Read the model definition and answer for the solid it produces. Units are mm, in the model's axes. A direction names the side the tool comes from. Round coordinates to 2 decimals unless told otherwise and drop trailing zeros. Order: outer loops, then holes, each group sorted by start corner. A loop starts at its lowest first (then second) coordinate and runs counter-clockwise, first axis right, second up. Notation, with made-up numbers: (-31.75, 49) - (5.25, 49) arc R22 cw to (5.25, 81) - close; hole circle Ø9 at (12.25, 43). An arc over 180 degrees is marked (long way). Put each result on its own line as item: value. Start each with the question number.
Q1. Section C-C on z = 36 is taken. Give the vertices of the cut face in (x, y).
Q2. Find the intervals of material crossed by line 1 along Y through (x, z) = (-19, 1.6); line 2 along X through (y, z) = (-7, 123); line 3 along X through (y, z) = (-7.25, 114.5), in increasing order. Write a range as from..to.
Q3. Each of these flat-tipped pins is pushed along its axis until it touches: pin 1 Ø9 at (y, z) = (-13, 81.5) entering from +X; pin 2 Ø5.5 at (x, z) = (0, 51.5) entering from +Y; pin 3 Ø1.5 at (x, y) = (-11, -15.5) entering from +Z; pin 4 Ø2.5 at (x, y) = (-19, -15) entering from -Z. Where does it stop, or does it pass through?
Q4. Which of the six approach directions +Z, -Z, +X, -X, +Y, -Y give full straight-line access (tool end or side, diameter ignored) to faces 1 (the face through (-9, -15, 6)), 2 (the face through (-0.05, -21.45, 100.94))?
Q5. Section B-B on y = -1.75 is taken. Give the vertices of the cut face in (x, z), then the cut area to 3 significant figures.
Q6. For a pull along X with two mould halves and no side action, classify faces 3 (the face through (9, -15, 7)), 4 (the face through (0, -14.279, 85)), 5 (the face through (1.85, -14.79, 126.33)) as pulls with the +X half, pulls with the -X half, needs draft (parallel to the pull), parting line crosses it, or undercut.
Q7. Section A-A on x = -19 is taken. Give the vertices of the cut face in (y, z).
Q8. Section D-D on x = 0 is taken. State how many separate pieces and enclosed holes the cut face has, then the cut area to 3 significant figures.
from build123d import *

# Parameters (mm, degrees)
F0_R     = 3.45
F1_DEPTH = 30
F2_R     = 1.5
F3_DEPTH = 25.4
F5_DEPTH = 25.4


with BuildPart() as f1:
    # F0 (on Front) → F1 (new body)
    with BuildSketch(Plane.XZ):
        Polygon((-24, 5), (-24, 0), (-9, 0), (-9, 13), (0, 13), (9, 13), (9, 0), (24, 0), (24, 5), (14, 5), (14, 18), (10.571068, 18), (3.5, 18), (0, 18), (-3.5, 18), (-10.571068, 18), (-14, 18), (-14, 5), align=None)
        Polygon((-3.5, 25.071068), (-10.571068, 18), (-3.5, 18), align=None)
        with BuildLine():
            Line((-3.5, 25.071068), (-3.5, 18))
            Line((-3.5, 18), (0, 18))
            Line((0, 18), (3.5, 18))
            Line((3.5, 18), (3.5, 25.071068))
            Line((3.5, 25.071068), (3.5, 118))
            ThreePointArc((3.5, 118), (0, 116.967795), (-3.5, 118))
            Line((-3.5, 118), (-3.5, 25.071068))
        make_face()
        with BuildLine():
            ThreePointArc((6.45, 123.417795), (-3.084437, 129.082488), (-3.5, 118))
            ThreePointArc((-3.5, 118), (0, 116.967795), (3.5, 118))
            ThreePointArc((3.5, 118), (5.664693, 120.333358), (6.45, 123.417795))
        make_face()
        with Locations((0, 123.417795)):
            Circle(F0_R, mode=Mode.SUBTRACT)
        Polygon((3.5, 25.071068), (3.5, 18), (10.571068, 18), align=None)
    extrude(amount=F1_DEPTH)

    # F2 (on face) → F3 (cut)
    with BuildSketch(Plane.XY.offset(5)):
        with Locations((19, -15)):
            Circle(F2_R)
        with Locations((-19, -15)):
            Circle(F2_R)
    extrude(amount=-F3_DEPTH, mode=Mode.SUBTRACT)

    # F4 (on face) → F5 (cut)
    with BuildSketch(Plane(origin=(-3.5, 0, 0), x_dir=(0, -1, 0), z_dir=(-1, 0, 0))):
        Polygon((14.351341, 41.974204), (4.138201, 34.047591), (14.351341, 34.047591), align=None)
        Polygon((4.138201, 38.620638), (14.351341, 46.547251), (4.138201, 46.852125), align=None)
        Polygon((14.351341, 57.451731), (4.138201, 49.525118), (14.351341, 49.525118), align=None)
        Polygon((4.138201, 54.098165), (14.351341, 62.024778), (4.138201, 62.329652), align=None)
        Polygon((14.279029, 73.874906), (4.065889, 65.948293), (14.279029, 65.948293), align=None)
        Polygon((4.065889, 70.52134), (14.279029, 78.447953), (4.065889, 78.752828), align=None)
        Polygon((14.279029, 89.352433), (4.065889, 81.42582), (14.279029, 81.42582), align=None)
        Polygon((4.065889, 85.998867), (14.279029, 93.92548), (4.065889, 94.230354), align=None)
        Polygon((26.558967, 41.64265), (16.345827, 33.716037), (26.558967, 33.716037), align=None)
        Polygon((16.345827, 38.289084), (26.558967, 46.215698), (16.345827, 46.520572), align=None)
        Polygon((26.558967, 57.120177), (16.345827, 49.193564), (26.558967, 49.193564), align=None)
        Polygon((16.345827, 53.766611), (26.558967, 61.693224), (16.345827, 61.998098), align=None)
        Polygon((26.486655, 73.543353), (16.273515, 65.61674), (26.486655, 65.61674), align=None)
        Polygon((16.273515, 70.189787), (26.486655, 78.1164), (16.273515, 78.421274), align=None)
        Polygon((26.486655, 89.02088), (16.273515, 81.094267), (26.486655, 81.094267), align=None)
        Polygon((16.273515, 85.667314), (26.486655, 93.593927), (16.273515, 93.898801), align=None)
        Polygon((14.279029, 105.178627), (4.065889, 97.252014), (14.279029, 97.252014), align=None)
        Polygon((4.065889, 101.825062), (14.279029, 109.751675), (4.065889, 110.056549), align=None)
        Polygon((26.486655, 104.847074), (16.273515, 96.920461), (26.486655, 96.920461), align=None)
        Polygon((16.273515, 101.493508), (26.486655, 109.420121), (16.273515, 109.724995), align=None)
    extrude(amount=-F5_DEPTH, mode=Mode.SUBTRACT)


solid = f1.part
Findings:
1. outline: (-3.5, -30) - (3.5, -30) - (3.5, -26.56) - (-3.5, -26.56) - close; (-3.5, -19.29) - (3.5, -19.29) - (3.5, -14.35) - (-3.5, -14.35) - close; (-3.5, -6.65) - (3.5, -6.65) - (3.5, 0) - (-3.5, 0) - close
2. line 1: -30..-16.5, -13.5..0
2. line 2: -6.44..-3.42, 3.42..6.44
2. line 3: -3.5..3.5
3. pin 1: x = 3.5
3. pin 2: y = 0
3. pin 3: z = 18.32
3. pin 4: through
4. face 1: -Z, +Y, -Y
4. face 2: +X, -X
5. outline: (-24, 0) - (-9, 0) - (-9, 13) - (9, 13) - (9, 0) - (24, 0) - (24, 5) - (14, 5) - (14, 18) - (10.57, 18) - (3.5, 25.07) - (3.5, 118) arc R6.45 ccw to (6.45, 123.42) arc R6.45 ccw (long way) to (-3.5, 118) - (-3.5, 25.07) - (-10.57, 18) - (-14, 18) - (-14, 5) - (-24, 5) - close; hole circle Ø6.9 at (0, 123.42)
5. area: 1,210 mm2
6. face 3: undercut
6. face 4: needs draft
6. face 5: undercut
7. outline: (-30, 0) - (-16.5, 0) - (-16.5, 5) - (-30, 5) - close; (-13.5, 0) - (0, 0) - (0, 5) - (-13.5, 5) - close
8. separate pieces: 2
8. enclosed holes: 20
8. area: 2,470 mm2
